```python
from build123d import *

# Parameters (mm, degrees)
SKETCH1_R           = 2.6
BOSS_EXTRUDE1_DEPTH = 5
SKETCH2_R           = 1.25
CUT_EXTRUDE1_DEPTH  = 2
SKETCH3_W           = 6
SKETCH3_H           = 3.7
CUT_EXTRUDE2_DEPTH  = 5


with BuildPart() as part:
    # Sketch1 → Boss-Extrude1 (new body)
    with BuildSketch(Plane.XY):
        with BuildLine():
            Line((-4.6, 0), (-4.6, 10))
            Line((-4.6, 10), (4.6, 10))
            Line((4.6, 10), (4.6, 0))
            ThreePointArc((4.6, 0), (0, -4.6), (-4.6, 0))
        make_face()
        Circle(SKETCH1_R, mode=Mode.SUBTRACT)
    extrude(amount=BOSS_EXTRUDE1_DEPTH)

    # Sketch2 → Cut-Extrude1 (cut)
    with BuildSketch(Plane(origin=(0, 10, 0), x_dir=(1, 0, 0), z_dir=(0, 1, 0))):
        with Locations(Location((0, -2.5, 0), (0, 0, 270))):
            Circle(SKETCH2_R)
    extrude(amount=-CUT_EXTRUDE1_DEPTH, mode=Mode.SUBTRACT)

    # Sketch3 → Cut-Extrude2 (cut)
    with BuildSketch(Plane.XY.offset(5)):
        with Locations((0, 6.15)):
            Rectangle(SKETCH3_W, SKETCH3_H)
    extrude(amount=-CUT_EXTRUDE2_DEPTH, mode=Mode.SUBTRACT)


solid = part.part
```
Part model, mm, in its own coordinate system. A direction names the side the tool comes from. Round coordinates to 2 decimals unless told otherwise and drop trailing zeros. Write each loop counter-clockwise with the first axis right and the second up, starting at its lowest first coordinate (ties: lowest second). Pieces come first, ordered by that corner, then holes.
Item 1: Cut at A-A, the plane y = 6.75. Give the cut face in (x, z).
Results:
outline: (-4.6, 0) - (-3, 0) - (-3, 5) - (-4.6, 5) - close; (3, 0) - (4.6, 0) - (4.6, 5) - (3, 5) - close
Item 2: Two-plate mould, pull along Y, no slides. Class faces 1 (the flat face through (-1, 10, 1)), 2 (the cylindrical face through (-0.338, 2.578, 2.465)), 3 (the flat face through (-4.6, 5, 2)): +Y half, -Y half, draft (parallel to the pull), parting line (faces both ways), or undercut.
Results:
face 1: +Y half
face 2: undercut
face 3: draft
Item 3: Drop flat-ended pins along their axis: pin 1 Ø3 at (x, y) = (0, 0) entering from +Z; pin 2 Ø3 at (x, z) = (0, 2.5) entering from +Y. Give the stop position or say it passes through.
Results:
pin 1: passes through
pin 2: stops at y = 10
Item 4: Cut at D-D, the plane z = 0.7. Give the cut face in (x, y), plus the area to 3 significant figures.
Results:
outline: (-4.6, 0) arc R4.6 ccw to (4.6, 0) - (4.6, 10) - (-4.6, 10) - close; hole (-3, 4.3) - (3, 4.3) - (3, 8) - (-3, 8) - close; hole circle Ø5.2 at (0, 0)
area: 81.8 mm2
Item 5: Cut at B-B, the plane z = 2.5. Give the cut face in (x, y).
Results:
outline: (-4.6, 0) arc R4.6 ccw to (4.6, 0) - (4.6, 10) - (1.25, 10) - (1.25, 8) - (3, 8) - (3, 4.3) - (-3, 4.3) - (-3, 8) - (-1.25, 8) - (-1.25, 10) - (-4.6, 10) - close; hole circle Ø5.2 at (0, 0)
Item 6: Probe L1, parallel to X at y = 8.4, z = 2.5; L2, parallel to Y at x = 1.25, z = 4.35; L3, parallel to Y at x = -1.75, z = 2.8. List the from-to ranges inside material, lowest first.
Results:
L1: x = -4.6 to -1.25, 1.25 to 4.6
L2: y = -4.43 to -2.28, 2.28 to 4.3, 8 to 10
L3: y = -4.25 to -1.92, 1.92 to 4.3, 8 to 10
Item 7: Cut at C-C, the plane x = 0. Give the cut face in (y, z), plus the area to 3 significant figures.
Results:
outline: (-4.6, 0) - (-2.6, 0) - (-2.6, 5) - (-4.6, 5) - close; (2.6, 0) - (4.3, 0) - (4.3, 5) - (2.6, 5) - close; (8, 0) - (10, 0) - (10, 1.25) - (8, 1.25) - close; (8, 3.75) - (10, 3.75) - (10, 5) - (8, 5) - close
area: 23.5 mm2
Item 8: Which spindle directions (+Z, -Z, +X, -X, +Y, -Y) get a long thin tool onto all of the face, cutting with end or side? Do faces 4 (the flat face through (-3, 6, 3)), 5 (the cylindrical face through (0.38, 9.01, 3.69)), 6 (the flat face through (4.6, 5, 2)). Say none if no direction does.
Results:
face 4: +Z, -Z
face 5: +Y
face 6: +Z, -Z, +X, +Y, -Y
